Source: CAD feature listing. Evaluate the final solid. Frame: model axes, mm. A direction names the side the tool comes from. Give positions to 0.01 mm unless a question says otherwise; leave off trailing zeros. Order: outer loops, then holes, each group sorted by start corner. A loop starts at its lowest first (then second) coordinate and runs counter-clockwise, first axis right, second up.
```python
from build123d import *

# Parameters (mm, degrees)
SKETCH1_R           = 2.3
BOSS_EXTRUDE2_DEPTH = 4
FILLET1_R           = 4
FILLET2_R           = 100
BOSS_EXTRUDE3_START = -5.575308
SKETCH2_R           = 2.3
BOSS_EXTRUDE3_DEPTH = 1.575308


with BuildPart() as part:
    # Sketch1 → Boss-Extrude2 (new body)
    with BuildSketch(Plane(origin=(0, 0, 0), x_dir=(1, 0, 0), z_dir=(0, 1, 0))):
        with BuildLine():
            Line((-4, -143.7), (-4, 4))
            Line((-4, 4), (25.4, 4))
            ThreePointArc((25.4, 4), (28.6800532, 2.289377864), (29.154640594, -1.379374498))
            Line((29.154640594, -1.379374498), (4, -69.85))
            Line((4, -69.85), (29.154640594, -138.320625502))
            ThreePointArc((29.154640594, -138.320625502), (28.6800532, -141.989377864), (25.4, -143.7))
            Line((25.4, -143.7), (-4, -143.7))
        make_face()
        with Locations(Location((0, 0, 0), (0, 0, 270))):
            Circle(SKETCH1_R, mode=Mode.SUBTRACT)
        with Locations(Location((25.4, 0, 0), (0, 0, 270))):
            Circle(SKETCH1_R, mode=Mode.SUBTRACT)
        with Locations(Location((25.4, -139.7, 0), (0, 0, 270))):
            Circle(SKETCH1_R, mode=Mode.SUBTRACT)
        with Locations(Location((0, -139.7, 0), (0, 0, 270))):
            Circle(SKETCH1_R, mode=Mode.SUBTRACT)
    extrude(amount=BOSS_EXTRUDE2_DEPTH)

    # Fillet1
    fillet1_edges = [part.edges().sort_by_distance(p)[0] for p in [
        (-4, 2, 143.7),
        (-4, 2, -4),
    ]]
    fillet(fillet1_edges, radius=FILLET1_R)

    # Fillet2
    fillet2_edges = [part.edges().sort_by_distance(p)[0] for p in [
        (4, 2, 69.85),
    ]]
    fillet(fillet2_edges, radius=FILLET2_R)

    # Sketch2 → Boss-Extrude3 (add)
    with BuildSketch(Plane(origin=(0, 4, 0), x_dir=(1, 0, 0), z_dir=(0, 1, 0)).offset(BOSS_EXTRUDE3_START)):
        with BuildLine():
            Line((0, -4), (25.4, -4))
            ThreePointArc((25.4, -4), (29.4, 0), (25.4, 4))
            Line((25.4, 4), (0, 4))
            ThreePointArc((0, 4), (-4, 0), (0, -4))
        make_face()
        with Locations(Location((0, 0, 0), (0, 0, 270))):
            Circle(SKETCH2_R, mode=Mode.SUBTRACT)
        with Locations(Location((25.4, 0, 0), (0, 0, 270))):
            Circle(SKETCH2_R, mode=Mode.SUBTRACT)
    extrude(amount=BOSS_EXTRUDE3_DEPTH)


solid = part.part
```
1) Reachability of faces 1 (the cylindrical face through (-3.73, 0.55, -1.45)), 2 (the flat face through (22.824, 1.972, 121.09)), 3 (the cylindrical face through (23.36, 1.17, 1.06)) from +Z, -Z, +X, -X, +Y, -Y: full face, straight path, thin tool, end or side. Return the list, or none.
Report:
face 1: -X, -Y
face 2: +X, +Y, -Y
face 3: +Y, -Y
2) Section query A-A, the plane x = 19.5. Return the cut outline in (y, z).
Report:
outline: (-1.58, -4) - (4, -4) - (4, 27.66) - (0, 27.66) - (0, 4) - (-1.58, 4) - close; (0, 112.04) - (4, 112.04) - (4, 143.7) - (0, 143.7) - close
3) Pin query (flat end, axial travel): pin 1 (10 mm diameter, centred on x = 12, z = 42.5, fed in from -Y); pin 2 (3 mm diameter, centred on y = 0.5, z = 118, fed in from +X); pin 3 (0.5 mm diameter, centred on x = 18, y = -1, fed in from +Z). Return the tip coordinate at first contact, or that it passes through.
Report:
pin 1: stops at y = 0
pin 2: stops at x = 22.24
pin 3: stops at z = 4
4) Section query C-C, the plane z = 91.5. Return the cut outline in (x, y).
Report:
outline: (-4, 0) - (12.91, 0) - (12.91, 4) - (-4, 4) - close
5) Material intervals for L1, parallel to X at y = 2.5, z = 0; L2, parallel to Z at x = -0.5, y = 2.9 (3 decimals); L3, parallel to X at y = 1, z = 138.5, sorted ascending.
Report:
L1: x = -4 to -2.3, 2.3 to 23.1, 27.7 to 29.4
L2: z = -3.969 to -2.245, 2.245 to 137.455, 141.945 to 143.669
L3: x = -4 to -1.96, 1.96 to 23.44, 27.36 to 29.22
6) Section query B-B, the plane z = 118. Return the cut outline in (x, y).
Report:
outline: (-4, 0) - (21.69, 0) - (21.69, 4) - (-4, 4) - close
